The model under review builds one solid part; all positions refer to its coordinate system, in mm. A direction names the side the tool comes from. Give positions to 0.01 mm unless a question says otherwise; leave off trailing zeros. Loops run counter-clockwise (first coordinate to the right, second up) from the corner with the lowest first, then second, coordinate; pieces in that order, holes last. Notation, with made-up numbers: (-27.5, 75.5) - (-0.5, 75.5) arc R12 ccw to (-0.5, 90.5) - close; hole circle Ø6 at (47, 53). An arc over 180 degrees is marked (long way). Answer as a JSON object with one key per item and string values.
from build123d import *

# Parameters (mm, degrees)
CROQUIS1_R              = 2.15
SALIENTE_EXTRUIR1_DEPTH = 20
REDONDEO1_R             = 20
CROQUIS4_R              = 2.15
CORTAR_EXTRUIR3_DEPTH   = 20
REDONDEO2_R             = 3


with BuildPart() as part:
    # Croquis1 → Saliente-Extruir1 (new body)
    with BuildSketch(Plane.XY):
        Polygon((-60, 0), (-11.715728753, 0), (60, -71.715728753), (60, -170), (40, -170), (40, -80), (-20, -20), (-60, -20), align=None)
        with Locations((-45, -10)):
            Circle(CROQUIS1_R, mode=Mode.SUBTRACT)
    extrude(amount=SALIENTE_EXTRUIR1_DEPTH)

    # Redondeo1
    redondeo1_edges = [part.edges().sort_by_distance(p)[0] for p in [
        (-20, -20, 10),
        (40, -80, 10),
        (60, -71.715728753, 10),
        (-11.715728753, 0, 10),
    ]]
    fillet(redondeo1_edges, radius=REDONDEO1_R)

    # Croquis4 → Cortar-Extruir3 (cut)
    with BuildSketch(Plane.ZY.offset(-40)):
        with Locations(Location((10, -155, 0), (0, 0, 270))):
            Circle(CROQUIS4_R)
    extrude(amount=-CORTAR_EXTRUIR3_DEPTH, mode=Mode.SUBTRACT)

    # Redondeo2
    redondeo2_edges = [part.edges().sort_by_distance(p)[0] for p in [
        (-40, 0, 0),
        (-60, -10, 0),
        (-60, -20, 10),
        (40, -170, 10),
        (60, -170, 10),
        (-60, 0, 10),
        (50, -170, 20),
        (40, -129.142135624, 20),
        (10, -50, 0),
        (10, -50, 20),
        (24.142135624, -35.857864376, 0),
        (24.142135624, -35.857864376, 20),
        (60, -125, 0),
        (-44.142135624, -20, 0),
        (-12.346331353, -1.52240935, 0),
        (58.47759065, -72.346331353, 0),
        (60, -125, 20),
        (-44.142135624, -20, 20),
        (-12.346331353, -1.52240935, 20),
        (58.47759065, -72.346331353, 20),
        (38.47759065, -80.6306026, 0),
        (38.47759065, -80.6306026, 20),
        (-20.6306026, -21.52240935, 0),
        (-20.6306026, -21.52240935, 20),
        (-60, -10, 20),
        (-40, 0, 20),
        (40, -129.142135624, 0),
        (50, -170, 0),
    ]]
    fillet(redondeo2_edges, radius=REDONDEO2_R)


solid = part.part
Q1. Consider section C-C, the plane x = -31. State the section outline as (y, z) points.
Results:
{"outline": "(-20, 3) arc R3 ccw to (-17, 0) - (-3, 0) arc R3 ccw to (0, 3) - (0, 17) arc R3 ccw to (-3, 20) - (-17, 20) arc R3 ccw to (-20, 17) - close"}
Q2. Clearance check with flat-ended pins moving along their axes: pin 1 Ø5 at (y, z) = (-155, 10) entering from +X; pin 2 Ø12 at (y, z) = (-66.5, 16.5) entering from -X; pin 3 Ø12 at (y, z) = (-56.5, 16) entering from +X; pin 4 Ø1 at (y, z) = (-18.5, 18) entering from -X. State where each tip first meets the part, or that it passes through.
Results:
{"pin 1": "stops at x = 60", "pin 2": "stops at x = 20.5", "pin 3": "stops at x = 50.78", "pin 4": "stops at x = -59.7"}
Q3. For faces 5 (the face through (40, -128, 10)), 6 (the face through (50, -170, 10)), list the 3-axis set-ups (+Z, -Z, +X, -X, +Y, -Y) from which the entire face can be reached by the end or side of a thin tool; tool diameter is ignored.
Results:
{"face 5": "+Z, -Z, -X, -Y", "face 6": "+Z, -Z, +X, -X, -Y"}
Q4. Consider section A-A, the plane z = 10. State the section outline as (x, y) points, plus the area to 3 significant figures.
Results:
{"outline": "(-60, -17) arc R3 ccw to (-57, -20) - (-28.28, -20) arc R20 cw to (-14.14, -25.86) - (34.14, -74.14) arc R20 cw to (40, -88.28) - (40, -152.85) - (60, -152.85) - (60, -80) arc R20 ccw to (54.14, -65.86) - (-5.86, -5.86) arc R20 ccw to (-20, 0) - (-57, 0) arc R3 ccw to (-60, -3) - close; (40, -167) arc R3 ccw to (43, -170) - (57, -170) arc R3 ccw to (60, -167) - (60, -157.15) - (40, -157.15) - close; hole circle Ø4.3 at (-45, -10)", "area": "4,520 mm^2"}
Q5. To check wall thickness, follow probe 1 along Z at (x, y) = (50.75, -155); probe 2 along Y at (x, z) = (-55, 10.75); probe 3 along X at (y, z) = (-129, 12.75). State the ranges of each line that lie inside material, in increasing order. Write a range as [from, to].
Results:
{"probe 1": "z = [0, 7.85], [12.15, 20]", "probe 2": "y = [-20, 0]", "probe 3": "x = [40, 60]"}
Q6. Consider section D-D, the plane x = -45. State the section outline as (y, z) points.
Results:
{"outline": "(-20, 3) arc R3 ccw to (-17, 0) - (-12.15, 0) - (-12.15, 20) - (-17, 20) arc R3 ccw to (-20, 17) - close; (-7.85, 0) - (-3, 0) arc R3 ccw to (0, 3) - (0, 17) arc R3 ccw to (-3, 20) - (-7.85, 20) - close"}
Q7. Consider section B-B, the plane y = -155. State the section outline as (x, z) points, plus the area to 3 significant figures.
Results:
{"outline": "(40, 3) arc R3 ccw to (43, 0) - (57, 0) arc R3 ccw to (60, 3) - (60, 7.85) - (40, 7.85) - close; (40, 12.15) - (60, 12.15) - (60, 17) arc R3 ccw to (57, 20) - (43, 20) arc R3 ccw to (40, 17) - close", "area": "306 mm^2"}
Q8. The part is to be moulded in two halves that separate along X. For faces 1 (the face through (-42, -20, 10)), 2 (the face through (23.957, -36.883, 0.902)), 3 (the face through (-20.73, -21.48, 10.1)), 4 (the face through (-42.95, -9.35, 9.86)), say which applies: +X half, -X half, draft (parallel to the pull), parting line (faces both ways), or undercut.
Results:
{"face 1": "draft", "face 2": "+X half", "face 3": "-X half", "face 4": "undercut"}
